Read the model definition and answer for the solid it produces. Units are mm, in the model's axes. Face numbers are marked on the shaded views. A direction names the side the tool comes from. Give positions to 0.01 mm unless a question says otherwise; leave off trailing zeros. Order: outer loops, then holes, each group sorted by start corner. A loop starts at its lowest first (then second) coordinate and runs counter-clockwise, first axis right, second up. Notation, with made-up numbers: M -24,43.5 L 24,43.5 A22 ccw 24,71.5 Z; hole C -27,40 d2. An arc over 180 degrees is marked long. One line per item, written item: value. Start each with the question number.
from build123d import *

# Parameters (mm, degrees)
F0_W      = 42
F0_H      = 42
F1_DEPTH  = 12.5
F2_R      = 1.5
F3_DEPTH  = 25.001
F6_R      = 17.4
F7_DEPTH  = 5
F8_DEPTH  = 4.6
F9_W      = 10
F9_H      = 7
F10_DEPTH = 24.5
F11_R     = 2.75
F12_DEPTH = 3


with BuildPart() as f1:
    # F0 (on Front) → F1 (new body, symmetric)
    with BuildSketch(Plane.XZ):
        Rectangle(F0_W, F0_H)
    extrude(amount=F1_DEPTH, both=True)

    # F2 (on face) → F3 (cut, through all)
    with BuildSketch(Plane.XZ.offset(12.5)):
        with Locations((-15.5, 15.5)):
            Circle(F2_R)
        with Locations((15.5, 15.5)):
            Circle(F2_R)
        with Locations((-15.5, -15.5)):
            Circle(F2_R)
        with Locations((15.5, -15.5)):
            Circle(F2_R)
    extrude(amount=-F3_DEPTH, mode=Mode.SUBTRACT)

    # F4 (on Front) → F5 (revolve, cut)
    with BuildSketch(Plane.XZ):
        Polygon((13.55, -8.3), (5.55, -8.3), (5.55, -21), (13.55, -21), (13.55, -18), (11.55, -18), (11.55, -12), (13.55, -12), align=None)
    revolve(axis=Axis((5.55, 0, -42.7623434187), (0, 0, -1)), mode=Mode.SUBTRACT)

    # F6 (on Front) → F7 (join)
    with BuildSketch(Plane.XZ):
        with Locations((15, 12)):
            Circle(F6_R)
    extrude(amount=-F7_DEPTH)

    # F8 (add): a face of the model
    f8_faces = [f1.faces().sort_by_distance(p)[0] for p in [
        (21, -0.3429519104, -1.1432103634),
    ]]
    extrude(f8_faces, amount=F8_DEPTH)

    # F9 (on face) → F10 (join)
    with BuildSketch(Plane.XY.offset(21)):
        with Locations((0.1083916248, 0)):
            Rectangle(F9_W, F9_H)
    extrude(amount=F10_DEPTH)

    # F11 (on face) → F12 (join)
    with BuildSketch(Plane.XZ.offset(12.5)):
        with Locations((-15.5, 15.5)):
            Circle(F11_R)
        with Locations((-15.5, -15.5)):
            Circle(F11_R)
        with Locations((15.5, -15.5)):
            Circle(F11_R)
        with Locations((15.5, 15.5)):
            Circle(F11_R)
    extrude(amount=F12_DEPTH)


solid = f1.part
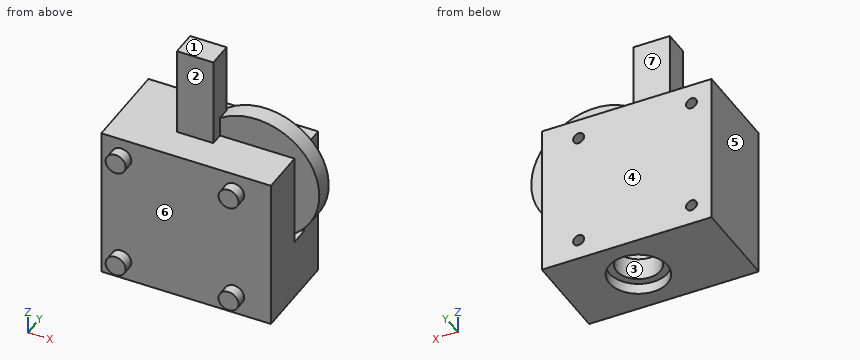
Q1. Each of these flat-tipped pins is pushed along its axis until it touches: pin 1 (0.9 mm diameter, centred on x = -15.5, z = 15, fed in from +Y); pin 2 (9.5 mm diameter, centred on x = 5.55, y = 0, fed in from +Z); pin 3 (2 mm diameter, centred on y = -1, z = 29.5, fed in from -X); pin 4 (8 mm diameter, centred on x = -5, z = 4.5, fed in from -Y). Where does it stop, or does it pass through?
Q2. Find section D-D, the plane x = 15. Give the vertices of the cut face in (y, z).
Q3. Consider probe 1 along Z at (x, y) = (-15.5, 4.5); probe 2 along Y at (x, z) = (5.55, -15.5); probe 3 along X at (y, z) = (0, -19.9). Determine where each line is inside the solid, lowest interval first.
Q4. A tool of negligible diameter and unlimited length cuts with its end or side. For the marked faces 5, 6 and 7, from which of +Z, -Z, +X, -X, +Y, -Y can it reach the whole face along a straight path? Write none if from no direction.
Q5. Find section C-C, the plane x = -3.5. Give the vertices of the cut face in (y, z).
Q6. Find section A-A, the plane z = -15.5. Give the vertices of the cut face in (x, y), then the cut area to 3 significant figures.
Q7. Find section B-B, the plane y = 9. Give the vertices of the cut face in (x, z), then the cut area to 3 significant figures.
Q8. Determine the mould class of the marked faces 1, 2, 3 and 4 for opening direction Y: released by +Y, released by -Y, zero draft, split by the parting line, or undercut.
Evaluation:
1. pin 1: y = -12.5
1. pin 2: z = 45.5
1. pin 3: x = -4.89
1. pin 4: y = -12.5
2. outline: M -15.5,-18.2 L -12.5,-18.2 L -12.5,-21 L 12.5,-21 L 12.5,-16.91 L -12.5,-16.91 L -12.5,-14.09 L 12.5,-14.09 L 12.5,14.09 L 5,14.09 L 5,16.91 L 12.5,16.91 L 12.5,21 L 5,21 L 5,29.4 L 0,29.4 L 0,21 L -12.5,21 L -12.5,18.2 L -15.5,18.2 L -15.5,12.8 L -12.5,12.8 L -12.5,-12.8 L -15.5,-12.8 Z; hole M -12.5,14.09 L 0,14.09 L 0,16.91 L -12.5,16.91 Z
3. probe 1: -21 to -17, -14 to 14, 17 to 21
3. probe 2: -12.5 to -6, 6 to 12.5
3. probe 3: -21 to -2.45, 13.55 to 25.6
4. face 5: +Z, -Z, -X, +Y, -Y
4. face 6: -Y
4. face 7: +Z, -X, +Y
5. outline: M -12.5,-21 L 12.5,-21 L 12.5,21 L 3.5,21 L 3.5,45.5 L -3.5,45.5 L -3.5,21 L -12.5,21 Z
6. outline: M -21,-12.5 L -18.25,-12.5 L -18.25,-15.5 L -12.75,-15.5 L -12.75,-12.5 L 12.75,-12.5 L 12.75,-15.5 L 18.25,-15.5 L 18.25,-12.5 L 25.6,-12.5 L 25.6,12.5 L 17,12.5 L 17,-12.5 L 14,-12.5 L 14,12.5 L -14,12.5 L -14,-12.5 L -17,-12.5 L -17,12.5 L -21,12.5 Z; hole C 5.55,0 d12
6. area: 935 mm2
7. outline: M -21,-21 L 25.6,-21 L 25.6,21 L -21,21 Z; hole C -15.5,-15.5 d3; hole C -15.5,15.5 d3; hole C 15.5,-15.5 d3; hole C 15.5,15.5 d3
7. area: 1,930 mm2
8. face 1: zero draft
8. face 2: released by -Y
8. face 3: undercut
8. face 4: released by +Y
